from build123d import *

# Parameters (mm, degrees)
F0_W     = 60.96
F0_H     = 63.5
F1_DEPTH = 6.35
F3_DEPTH = 6.351
F6_DEPTH = 6.351
F7_W     = 39.5752452314
F7_H     = 11.9200152457
F8_DEPTH = 6.351


# Not quite as in the source:
# - a feature of the source that left no trace in its solid (it failed there, or was rolled back) is left out


with BuildPart() as f1:
    # F0 (on Right) → F1 (new body)
    with BuildSketch(Plane.YZ):
        Rectangle(F0_W, F0_H)
    extrude(amount=F1_DEPTH)

    # F2 (on face) → F3 (cut, through all)
    with BuildSketch(Plane.YZ.offset(6.35)):
        with BuildLine():
            ThreePointArc((-3.81, 15.0182534271), (-9.5139869666, -12.2289855671), (15.494, 0))
            ThreePointArc((15.494, 0), (12.2289855671, 9.5139869666), (3.81, 15.0182534271))
            Line((3.81, 15.0182534271), (-3.81, 15.0182534271))
        make_face()
        with BuildLine():
            Line((-3.81, 15.0182534271), (3.81, 15.0182534271))
            ThreePointArc((3.81, 15.0182534271), (0, 15.494), (-3.81, 15.0182534271))
        make_face()
        with BuildLine():
            ThreePointArc((-3.81, 15.0182534271), (0, 15.494), (3.81, 15.0182534271))
            Line((3.81, 15.0182534271), (3.81, 24.1368534271))
            Line((3.81, 24.1368534271), (-3.81, 24.1368534271))
            Line((-3.81, 24.1368534271), (-3.81, 15.0182534271))
        make_face()
    extrude(amount=-F3_DEPTH, mode=Mode.SUBTRACT)

    # F5 (on face) → F6 (cut, through all)
    with BuildSketch(Plane.YZ.offset(6.35)):
        Polygon((30.48, 31.75), (-30.48, 31.75), (-30.48, 23.876), (-3.81, 23.876), (-3.81, 24.1368534271), (3.81, 24.1368534271), (3.81, 23.876), (30.48, 23.876), align=None)
    extrude(amount=-F6_DEPTH, mode=Mode.SUBTRACT)

    # F7 (on face) → F8 (cut, through all)
    with BuildSketch(Plane.YZ.offset(6.35)):
        Polygon((-19.7760853916, 23.876), (-30.48, 23.876), (-30.48, -31.75), (-19.7760853916, -31.75), (-19.7760853916, -19.8299847543), align=None)
        Polygon((19.7991598397, 23.876), (19.7991598397, -19.8299847543), (19.7991598397, -31.75), (30.48, -31.75), (30.48, 23.876), align=None)
        with Locations((0.0115372241, -25.7899923772)):
            Rectangle(F7_W, F7_H)
    extrude(amount=-F8_DEPTH, mode=Mode.SUBTRACT)


solid = f1.part
Can you work these out from the model? Positions are in its coordinate system, mm. Give positions to 0.01 mm unless a question says otherwise; leave off trailing zeros. Write each loop counter-clockwise with the first axis right and the second up, starting at its lowest first coordinate (ties: lowest second). Pieces come first, ordered by that corner, then holes. Notation, with made-up numbers: (14, 40.5) -> (72, 40.5) arc R24 cw to (72, 52.5) -> close; hole circle Ø6 at (36, -24.5). An arc over 180 degrees is marked (long way). Answer as a JSON object with one key per item and string values. Group by question number.
Item 1: Suppose I cut it at D-D (y = 0). Please give me the cut outline in (x, z), plus the area to 3 significant figures.
Item 2: We'd pull the mould along Y, two halves only. Please class faces 1 (the face through (3, -3.81, 20)), 2 (the face through (3, 12, 23.876)), 3 (the face through (3, 3.81, 19)), 4 (the face through (3, -19.776, 2)): +Y half, -Y half, draft (parallel to the pull), parting line (faces both ways), or undercut.
Item 3: I'm going to push a flat-ended pin straight in: P1, Ø1, axis at y = -15, z = -13, coming from the -X side. Where does the tip first touch, or does it pass through?
Item 4: Suppose I cut it at A-A (z = 20). Please give me the cut outline in (x, y), plus the area to 3 significant figures.
Item 5: Suppose I cut it at B-B (y = 15). Please give me the cut outline in (x, z), plus the area to 3 significant figures.
Item 6: Please list where these lines run through material, in increasing order: line 1 (Y direction, x = 4.75, z = 18); line 2 (Z direction, x = 4.25, y = 0); line 3 (Z direction, x = 1.25, y = -4.5). Write a range as [from, to].
Item 7: Suppose I cut it at C-C (x = 5). Please give me the cut outline in (y, z).
Findings:
{
 "1": {"outline": "(0, -19.83) -> (6.35, -19.83) -> (6.35, -15.49) -> (0, -15.49) -> close", "area": "27.5 mm²"},
 "2": {"face 1": "undercut", "face 2": "draft", "face 3": "undercut", "face 4": "-Y half"},
 "3": {"P1": "stops at x = 0"},
 "4": {"outline": "(0, -19.78) -> (6.35, -19.78) -> (6.35, -3.81) -> (0, -3.81) -> close; (0, 3.81) -> (6.35, 3.81) -> (6.35, 19.8) -> (0, 19.8) -> close", "area": "203 mm²"},
 "5": {"outline": "(0, -19.83) -> (6.35, -19.83) -> (6.35, -3.88) -> (0, -3.88) -> close; (0, 3.88) -> (6.35, 3.88) -> (6.35, 23.88) -> (0, 23.88) -> close", "area": "228 mm²"},
 "6": {"line 1": "y = [-19.78, -3.81], [3.81, 19.8]", "line 2": "z = [-19.83, -15.49]", "line 3": "z = [-19.83, -14.83], [14.83, 23.88]"},
 "7": {"outline": "(-19.78, -19.83) -> (19.8, -19.83) -> (19.8, 23.88) -> (3.81, 23.88) -> (3.81, 15.02) arc R15.49 cw (long way) to (-3.81, 15.02) -> (-3.81, 23.88) -> (-19.78, 23.88) -> close"}
}
